The model under review builds one solid part; all positions refer to its coordinate system, in mm. Face numbers are marked on the shaded views. Round coordinates to 2 decimals unless told otherwise and drop trailing zeros. Loops run counter-clockwise (first coordinate to the right, second up) from the corner with the lowest first, then second, coordinate; pieces in that order, holes last. Notation, with made-up numbers: M -10.75,-19 L 32.25,-19 A32 cw 32.25,12 Z; hole C -18.75,39 d5. An arc over 180 degrees is marked long. One line per question, with ' | ' between items.
from build123d import *

# Parameters (mm, degrees)
SKETCH1_R           = 8
BASEHEAD_DEPTH      = 10
SKETCH2_R           = 5
BASEBODY_DEPTH      = 90
HEXAGONSOCKET_DEPTH = 5
TOPFILLET_R         = 1.25
CHAMFER1_SIZE       = 0.4


with BuildPart() as part:
    # Sketch1 → BaseHead (new body)
    with BuildSketch(Plane(origin=(0, 0, 0), x_dir=(0, 0, -1), z_dir=(1, 0, 0))):
        Circle(SKETCH1_R)
    extrude(amount=BASEHEAD_DEPTH)

    # Sketch2 → BaseBody (add)
    with BuildSketch(Plane(origin=(10, 0, 0), x_dir=(0, 0, -1), z_dir=(1, 0, 0))):
        with Locations(Location((0, 0, 0), (0, 0, 180))):
            Circle(SKETCH2_R)
    extrude(amount=BASEBODY_DEPTH)

    # Sketch3 → HexagonSocket (cut)
    with BuildSketch(Plane(origin=(0, 0, 0), x_dir=(0, 0, -1), z_dir=(1, 0, 0))):
        Polygon((4.618802154, 0), (2.309401077, 4), (-2.309401077, 4), (-4.618802154, 0), (-2.309401077, -4), (2.309401077, -4), align=None)
    extrude(amount=HEXAGONSOCKET_DEPTH, mode=Mode.SUBTRACT)

    # Sketch4 → Cut-Revolve1 (revolve, cut)
    with BuildSketch(Plane(origin=(-4.19613823, 0.75, 0), x_dir=(-1, 0, 0), z_dir=(0, 0, 1)), mode=Mode.PRIVATE) as cut_revolve1_sk:
        Polygon((-9.19613823, 4.75), (-11.505539306, 0.75), (-9.19613823, 0.75), align=None)
    revolve(cut_revolve1_sk.sketch.rotate(Axis((0.838992387, 0, 0), (-1, 0, 0)), 90), axis=Axis((0.838992387, 0, 0), (-1, 0, 0)), mode=Mode.SUBTRACT)

    # TopFillet
    topfillet_edges = [part.edges().sort_by_distance(p)[0] for p in [
        (0, 0, 8),
    ]]
    fillet(topfillet_edges, radius=TOPFILLET_R)

    # Chamfer1
    chamfer1_edges = [part.edges().sort_by_distance(p)[0] for p in [
        (100, 0, -5),
    ]]
    chamfer(chamfer1_edges, length=CHAMFER1_SIZE)


solid = part.part
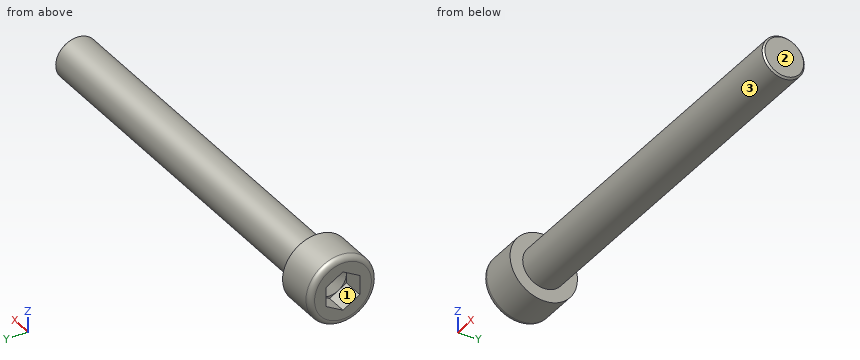
1) Add section A-A on x = 47. State the section outline as (y, z) points, then the cut area to 3 significant figures.
Output values:
outline: C 0,0 d10 | area: 78.5 mm²
2) For line 1 (X direction, y = 5, z = -3.5); line 2 (Z direction, x = 8.5, y = -6.25); line 3 (X direction, y = -3.75, z = 2), list the stretches that pass through material, from the lowest coordinate up.
Output values:
line 1: x = 0 to 10 | line 2: z = -4.99 to 4.99 | line 3: x = 5 to 100
3) Mouldability with a two-part tool opening along Z and no side actions: class the marked faces 1, 2 and 3 as +Z half, -Z half, draft (parallel to the pull), parting line (faces both ways), or undercut.
Output values:
face 1: undercut | face 2: draft | face 3: parting line
4) Insertion check: P1, Ø6, axis at x = 40, y = 1.5, coming from the +Z side; P2, Ø0.6, axis at y = 2.5, z = 2, coming from the -X side; P3, Ø5, axis at x = 89.5, z = 2.5, coming from the +Y side; P4, Ø1, axis at y = 5.5, z = -1, coming from the -X side. Each pin has a flat end and moves straight along its axis. Give the tip position at first contact, or say it passes through.
Output values:
P1: stops at z = 5 | P2: stops at x = 5.29 | P3: stops at y = 5 | P4: stops at x = 0
